from build123d import *

# Parameters (mm, degrees)
F1_DEPTH = 76.2
F3_DEPTH = 25.4


with BuildPart() as f1:
    # F0 (on Front) → F1 (new body)
    with BuildSketch(Plane.XZ):
        Polygon((-75.97407, 0), (0, 0), (76.292614, 0), (75.974077, 75.49423), (-75.97407, 75.814128), align=None)
        Polygon((76.292614, 0), (0, 0), (-75.97407, 0), (-75.97407, -76.134019), (76.613851, -76.134019), align=None)
    extrude(amount=F1_DEPTH)

    # F2 (on face) → F3 (join)
    with BuildSketch(Plane.XZ.offset(76.2)):
        Polygon((75.974077, 75.49423), (0, 0), (76.291256, 0.3219), align=None)
    extrude(amount=F3_DEPTH)


solid = f1.part
Geometry check sheet. Reference: the model listing, model coordinates, mm. A direction names the side the tool comes from. Give positions to 0.01 mm unless a question says otherwise; leave off trailing zeros. Write each loop counter-clockwise with the first axis right and the second up, starting at its lowest first coordinate (ties: lowest second). Pieces come first, ordered by that corner, then holes.
1) Go/stop test with flat-tipped pins: pin 1 Ø5 at (x, z) = (-24.5, 14) entering from -Y; pin 2 Ø12 at (y, z) = (-11.5, 59) entering from +X. Record where each tip stops, or that it passes through.
Values follow:
pin 1: stops at y = -76.2
pin 2: stops at x = 76.07
2) Thickness scan on line 1 (Y direction, x = 7, z = 34.5); line 2 (Z direction, x = 60, y = -19); line 3 (X direction, y = -10, z = -67). Record the ranges inside material, lowest first.
Values follow:
line 1: y = -76.2 to 0
line 2: z = -76.13 to 75.53
line 3: x = -75.97 to 76.58
3) Cross-section at A-A (x = 26.5). Record the boundary of the cut face in (y, z), plus the area to 3 significant figures.
Values follow:
outline: (-101.6, 0.11) - (-76.2, 0.11) - (-76.2, -76.13) - (0, -76.13) - (0, 75.6) - (-76.2, 75.6) - (-76.2, 26.33) - (-101.6, 26.33) - close
area: 12,200 mm2
4) Set-up check for faces 1 (the face through (38.519, -88.722, 38.276)), 2 (the face through (55, -101.6, 21)): record each of +Z, -Z, +X, -X, +Y, -Y from which the full face is reachable in a straight line by a thin tool's end or side.
Values follow:
face 1: +Z, -X, -Y
face 2: +Z, -Z, +X, -X, -Y
5) Cross-section at D-D (x = 52). Record the boundary of the cut face in (y, z).
Values follow:
outline: (-101.6, 0.22) - (-76.2, 0.22) - (-76.2, -76.13) - (0, -76.13) - (0, 75.54) - (-76.2, 75.54) - (-76.2, 51.67) - (-101.6, 51.67) - close
6) Cross-section at B-B (z = 29). Record the boundary of the cut face in (x, y), plus the area to 3 significant figures.
Values follow:
outline: (-75.97, -76.2) - (29.18, -76.2) - (29.18, -101.6) - (76.17, -101.6) - (76.17, 0) - (-75.97, 0) - close
area: 12,800 mm2
7) Cross-section at C-C (y = -80.5). Record the boundary of the cut face in (x, z), plus the area to 3 significant figures.
Values follow:
outline: (0, 0) - (76.29, 0.32) - (75.97, 75.49) - close
area: 2,870 mm2
